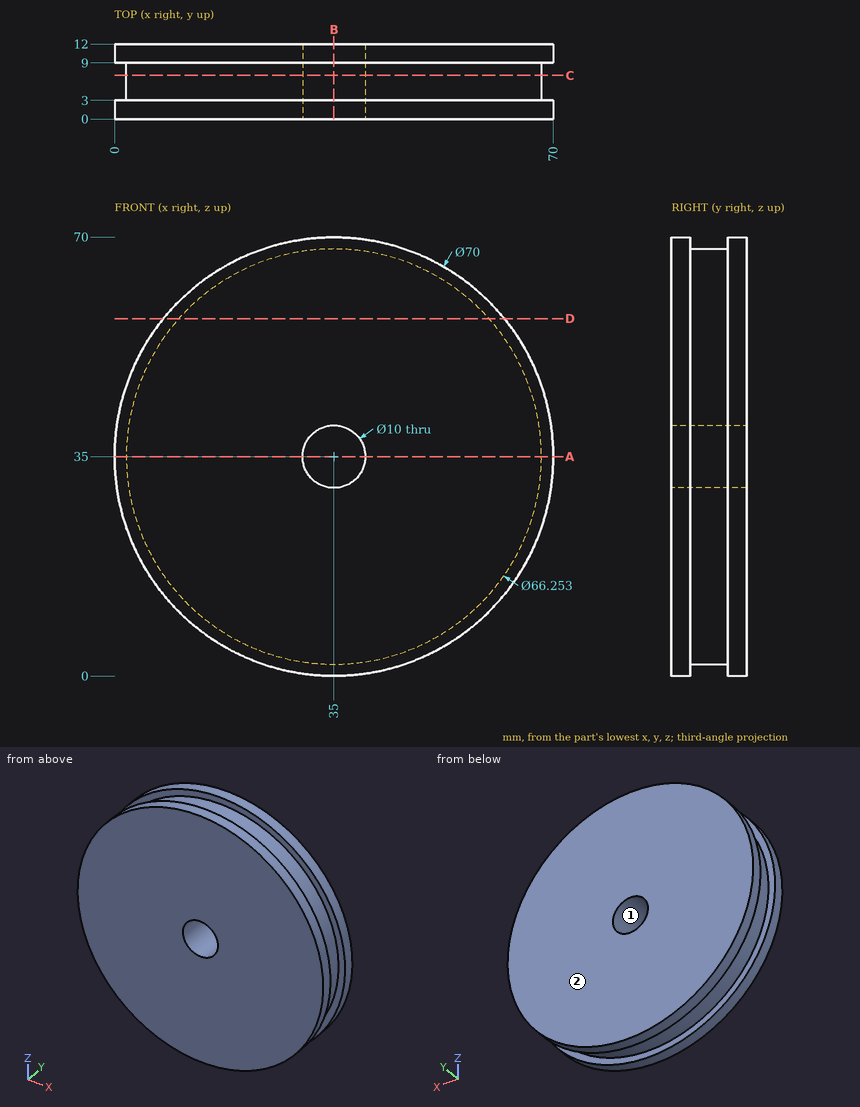
Geometry check sheet. Reference: drawing and pictorial views, mm from the part's lowest x, y, z. Round coordinates to 2 decimals unless told otherwise and drop trailing zeros. Write each loop counter-clockwise with the first axis right and the second up, starting at its lowest first coordinate (ties: lowest second). Pieces come first, ordered by that corner, then holes.
Item 1: Material ranges on line 1 along X through (y, z) = (3.25, 35); line 2 along Z through (x, y) = (65.5, 8); line 3 along Z through (x, y) = (18, 1.75), recorded low to high.
Determined:
line 1: x = 1.87 to 30, 40 to 68.13
line 2: z = 22.07 to 47.93
line 3: z = 4.41 to 65.59
Item 2: Mould release check, pull along Z, two halves, no side actions. Record for the marked faces 1 and 2: +Z half, -Z half, draft (parallel to the pull), parting line (faces both ways), or undercut.
Determined:
face 1: undercut
face 2: draft
Item 3: Section check D-D (z = 57). Record the boundary of the cut face in (x, y), plus the area to 3 significant figures.
Determined:
outline: (7.78, 0) - (62.22, 0) - (62.22, 3) - (59.77, 3) - (59.77, 9) - (62.22, 9) - (62.22, 12) - (7.78, 12) - (7.78, 9) - (10.23, 9) - (10.23, 3) - (7.78, 3) - close
area: 624 mm2
Item 4: Section check C-C (y = 7). Record the boundary of the cut face in (x, z), plus the area to 3 significant figures.
Determined:
outline: circle Ø66.25 at (35, 35); hole circle Ø10 at (35, 35)
area: 3,370 mm2
Item 5: Section check B-B (x = 35). Record the boundary of the cut face in (y, z).
Determined:
outline: (0, 0) - (3, 0) - (3, 1.87) - (9, 1.87) - (9, 0) - (12, 0) - (12, 30) - (0, 30) - close; (0, 40) - (12, 40) - (12, 70) - (9, 70) - (9, 68.13) - (3, 68.13) - (3, 70) - (0, 70) - close
Item 6: Go/stop test with flat-tipped pins: pin 1 Ø6 at (x, y) = (45.5, 2) entering from +Z; pin 2 Ø1.5 at (x, z) = (53.5, 53.5) entering from -Y. Record where each tip stops, or that it passes through.
Determined:
pin 1: stops at z = 69.19
pin 2: stops at y = 0
Item 7: Section check A-A (z = 35). Record the boundary of the cut face in (x, y).
Determined:
outline: (0, 0) - (30, 0) - (30, 12) - (0, 12) - (0, 9) - (1.87, 9) - (1.87, 3) - (0, 3) - close; (40, 0) - (70, 0) - (70, 3) - (68.13, 3) - (68.13, 9) - (70, 9) - (70, 12) - (40, 12) - close
